For this review, use the dimensioned drawing (mm, ordinates from the lowest corner) and the shaded views. A direction names the side the tool comes from. Round coordinates to 2 decimals unless told otherwise and drop trailing zeros. Write each loop counter-clockwise with the first axis right and the second up, starting at its lowest first coordinate (ties: lowest second). Pieces come first, ordered by that corner, then holes.
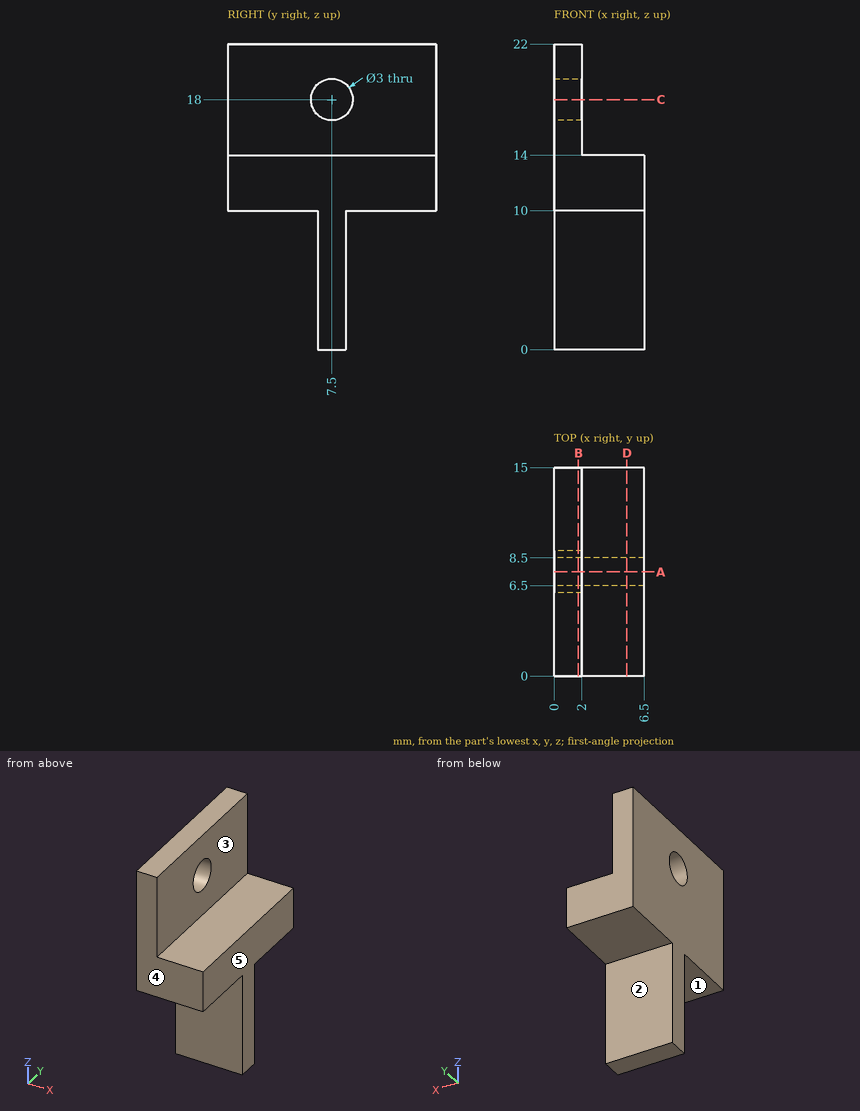
1) For the marked faces 1, 2, 3, 4 and 5, list the 3-axis set-ups (+Z, -Z, +X, -X, +Y, -Y) from which the entire face can be reached by the end or side of a thin tool; tool diameter is ignored.
2) For line 1 along Y through (x, z) = (0.7, 18); line 2 along Z through (x, y) = (2.5, 3.75); line 3 along Z through (x, y) = (1, 10.5), list the stretches that pass through material, from the lowest coordinate up.
3) Add section D-D on x = 5.25. State the section outline as (y, z) points, and give its area (3 significant figures).
4) Add section C-C on z = 18. State the section outline as (x, y) points, and give its area (3 significant figures).
5) Add section A-A on y = 7.5. State the section outline as (x, z) points, and give its area (3 significant figures).
6) Add section B-B on x = 1.75. State the section outline as (y, z) points, and give its area (3 significant figures).
7) For P1, Ø3, axis at x = 4.5, y = 10.5, coming from the -Z side; P2, Ø1.3, axis at x = 4.5, y = 9.5, coming from the +Z side; P3, Ø3, axis at x = 2, z = 6, coming from the +Y side, all flat-tipped, find the tip position at first contact; note any pin that passes through.
Computed:
1. face 1: -Z, +X, -X, -Y
1. face 2: -Z, +X, -X, +Y
1. face 3: +Z, +X, +Y, -Y
1. face 4: +Z, -Z, +X, -X, -Y
1. face 5: +Z, -Z, +X, +Y, -Y
2. line 1: y = 0 to 6, 9 to 15
2. line 2: z = 10 to 14
2. line 3: z = 10 to 22
3. outline: (0, 10) - (6.5, 10) - (6.5, 0) - (8.5, 0) - (8.5, 10) - (15, 10) - (15, 14) - (0, 14) - close
3. area: 80.0 mm2
4. outline: (0, 0) - (2, 0) - (2, 6) - (0, 6) - close; (0, 9) - (2, 9) - (2, 15) - (0, 15) - close
4. area: 24.0 mm2
5. outline: (0, 0) - (6.5, 0) - (6.5, 14) - (2, 14) - (2, 16.5) - (0, 16.5) - close; (0, 19.5) - (2, 19.5) - (2, 22) - (0, 22) - close
5. area: 101 mm2
6. outline: (0, 10) - (6.5, 10) - (6.5, 0) - (8.5, 0) - (8.5, 10) - (15, 10) - (15, 22) - (0, 22) - close; hole circle Ø3 at (7.5, 18)
6. area: 193 mm2
7. P1: stops at z = 10
7. P2: stops at z = 14
7. P3: stops at y = 8.5
